from build123d import *

# Parameters (mm, degrees)
F0_R     = 73.66
F0_R_2   = 10
F1_DEPTH = 15
F2_R     = 1
F3_DEPTH = 25
F4_R     = 5


with BuildPart() as f1:
    # F0 (on Front) → F1 (new body)
    with BuildSketch(Plane.XZ):
        Circle(F0_R)
        with Locations((-31.269082, -43.038199)):
            Circle(F0_R_2, mode=Mode.SUBTRACT)
        with Locations((0, -53.19814)):
            Circle(F0_R_2, mode=Mode.SUBTRACT)
        with Locations((-50.594438, -16.439129)):
            Circle(F0_R_2, mode=Mode.SUBTRACT)
        with Locations((31.269082, -43.038199)):
            Circle(F0_R_2, mode=Mode.SUBTRACT)
        with Locations((50.594438, -16.439129)):
            Circle(F0_R_2, mode=Mode.SUBTRACT)
        with Locations((-50.594438, 16.439129)):
            Circle(F0_R_2, mode=Mode.SUBTRACT)
        with Locations((-31.269082, 43.038199)):
            Circle(F0_R_2, mode=Mode.SUBTRACT)
        with Locations((0, 53.19814)):
            Circle(F0_R_2, mode=Mode.SUBTRACT)
        with Locations((50.594438, 16.439129)):
            Circle(F0_R_2, mode=Mode.SUBTRACT)
        with Locations((31.269082, 43.038199)):
            Circle(F0_R_2, mode=Mode.SUBTRACT)
    extrude(amount=F1_DEPTH)

    # F2 (on Front) → F3 (cut)
    with BuildSketch(Plane.XZ):
        Circle(F2_R)
    extrude(amount=F3_DEPTH, mode=Mode.SUBTRACT)

    # F4
    f4_edges = [f1.edges().sort_by_distance(p)[0] for p in [
        (-73.66, -15, 0),
        (-73.66, 0, 0),
    ]]
    fillet(f4_edges, radius=F4_R)


solid = f1.part
Model file for the job. Use its own axes, mm. Give positions to 0.01 mm unless a question says otherwise; leave off trailing zeros. One line per item, written item: value.
Item 1: Wall check: line 1 (X direction, y = -10, z = -14.5); line 2 (X direction, y = -9, z = 22); line 3 (Z direction, x = -2, y = -4.25). Give the ranges that are in metal, low to high.
Response values:
line 1: -72.22 to -60.4, -40.78 to 40.78, 60.4 to 72.22
line 2: -70.3 to -58.91, -42.28 to 42.28, 58.91 to 70.3
line 3: -73.58 to -63, -43.4 to 43.4, 63 to 73.58
Item 2: Two-plate mould, pull along X, no slides. Class faces 1 (the cylindrical face through (-58.454, -7.465, -44.821)), 2 (the cylindrical face through (43.224, -7.395, 23.198)), 3 (the cylindrical face through (40.81, -7.4, 46.04)), 4 (the flat face through (-1, -15, 1)): released by +X, released by -X, zero draft, split by the parting line, or undercut.
Response values:
face 1: split by the parting line
face 2: undercut
face 3: undercut
face 4: zero draft
Item 3: Slice it at A-A (y = -12.75). Give the number of separate pieces and of enclosed holes in the cut face, then the cut area to 3 significant figures.
Response values:
separate pieces: 1
enclosed holes: 11
area: 13,500 mm2
Item 4: Pin check, flat tips, straight feed: pin 1 Ø6 at (x, y) = (22, -7) entering from +Z; pin 2 Ø6 at (x, y) = (-44, -12.5) entering from +Z; pin 3 Ø4 at (x, z) = (-20.5, -54) entering from +Y; pin 4 Ø6 at (x, y) = (-1, -11) entering from -Z. Stop position of each tip, or through.
Response values:
pin 1: z = 71.17
pin 2: z = 60.82
pin 3: y = 0
pin 4: z = -73.66
